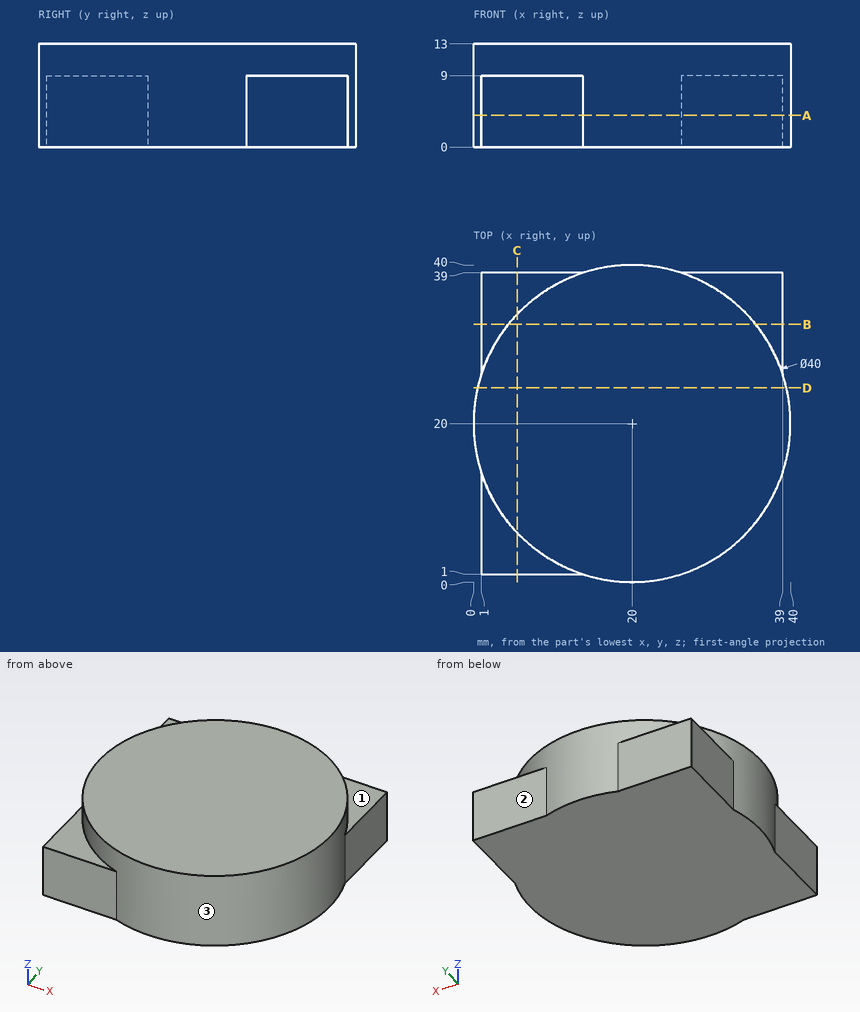
Part print with two shaded views. Sizes in mm from the minimum x, y, z corner. A direction names the side the tool comes from. Round coordinates to 2 decimals unless told otherwise and drop trailing zeros. Loops run counter-clockwise (first coordinate to the right, second up) from the corner with the lowest first, then second, coordinate; pieces in that order, holes last. Notation, with made-up numbers: M 39,77.25 L 79,77.25 A26 ccw 79,91.25 Z; hole C -8,10.25 d3. An arc over 180 degrees is marked long. Return JSON: item names as keys, results as strings. Group by question number.
(1) Tool access for the marked faces 1, 2 and 3: list every direction of +Z, -Z, +X, -X, +Y, -Y with a clear straight run to the whole face (end or side of a thin tool).
(2) Drop flat-ended pins along their axis: P1, Ø4, axis at y = 35, z = 8.5, coming from the -X side; P2, Ø3, axis at y = 14.5, z = 10.5, coming from the +X side; P3, Ø5, axis at y = 34.5, z = 3, coming from the +X side. Give the stop position or say it passes through.
(3) Wall check: probe 1 along Y at (x, z) = (6, 7.5); probe 2 along X at (y, z) = (20.5, 10.75). Give the ranges that are in metal, low to high. Write a range as [from, to].
(4) Saw through at C-C, the plane x = 5.5. List the corners of the cut face in (y, z).
(5) Saw through at B-B, the plane y = 32.5. List the corners of the cut face in (x, z).
(6) Saw through at A-A, the plane z = 4. List the corners of the cut face in (x, y) (3 decimals).
(7) Saw through at D-D, the plane y = 24.5. List the corners of the cut face in (x, z).
Answer list:
{
 "1": {"face 1": "+Z, +X, +Y", "face 2": "+Z, -Z, +X, +Y", "face 3": "+Z"},
 "2": {"P1": "x = 1", "P2": "x = 39.6", "P3": "x = 39"},
 "3": {"probe 1": "[1, 39]", "probe 2": "[0.01, 39.99]"},
 "4": {"outline": "M 1,0 L 39,0 L 39,9 L 33.77,9 L 33.77,13 L 6.23,13 L 6.23,9 L 1,9 Z"},
 "5": {"outline": "M 1,0 L 39,0 L 39,9 L 35.61,9 L 35.61,13 L 4.39,13 L 4.39,9 L 1,9 Z"},
 "6": {"outline": "M 1,1 L 13.755,1 A20 ccw 39,26.245 L 39,39 L 26.245,39 A20 ccw 13.755,39 L 1,39 L 1,26.245 A20 ccw 1,13.755 Z"},
 "7": {"outline": "M 0.51,0 L 39.49,0 L 39.49,13 L 0.51,13 Z"}
}
